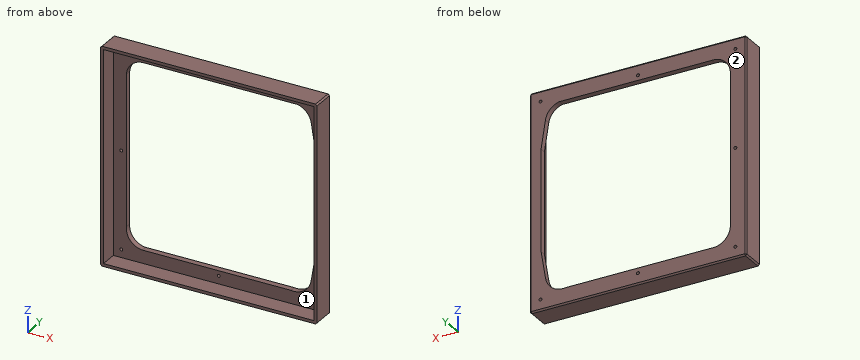
from build123d import *

# Parameters (mm, degrees)
SKETCH009_W     = 150
SKETCH009_H     = 150
SKETCH009_W_2   = 146
SKETCH009_H_2   = 146
PAD003_DEPTH    = 12
SKETCH010_W     = 150
SKETCH010_H     = 150
SKETCH010_R     = 1
PAD004_DEPTH    = 4
CHAMFER003_SIZE = 1


with BuildPart() as part:
    # Sketch009 → Pad003 (new body)
    with BuildSketch(Plane.XZ):
        Rectangle(SKETCH009_W, SKETCH009_H)
        Rectangle(SKETCH009_W_2, SKETCH009_H_2, mode=Mode.SUBTRACT)
    extrude(amount=PAD003_DEPTH)

    # Sketch010 (on Face9 of Pad003) → Pad004 (join)
    with BuildSketch(Plane(origin=(0, 0, 0), x_dir=(1, 0, 0), z_dir=(0, 1, 0))):
        Rectangle(SKETCH010_W, SKETCH010_H)
        with Locations((-67.5, 67.5)):
            Circle(SKETCH010_R, mode=Mode.SUBTRACT)
        with Locations((67.5, 67.5)):
            Circle(SKETCH010_R, mode=Mode.SUBTRACT)
        with Locations((0, 67.5)):
            Circle(SKETCH010_R, mode=Mode.SUBTRACT)
        with Locations((-67.5, 0)):
            Circle(SKETCH010_R, mode=Mode.SUBTRACT)
        with Locations((-67.5, -67.5)):
            Circle(SKETCH010_R, mode=Mode.SUBTRACT)
        with Locations((0, -67.5)):
            Circle(SKETCH010_R, mode=Mode.SUBTRACT)
        with Locations((67.5, -67.5)):
            Circle(SKETCH010_R, mode=Mode.SUBTRACT)
        with BuildLine():
            ThreePointArc((-53, 64), (-61.176409, 59.816751), (-64, 51.077152))
            Line((-64, 51.077152), (-64, -53))
            ThreePointArc((-64, -53), (-59.816751, -61.176409), (-51.077152, -64))
            Line((-51.077152, -64), (54.6127, -64))
            ThreePointArc((54.6127, -64), (60.907852, -60.466964), (64.115604, -54))
            Line((67.115604, -35), (64.115604, -54))
            Line((67.115604, 35), (67.115604, -35))
            Line((64, 54), (67.115604, 35))
            ThreePointArc((64, 54), (59.109644, 61.883516), (50.077152, 64))
            Line((50.077152, 64), (-53, 64))
        make_face(mode=Mode.SUBTRACT)
    extrude(amount=PAD004_DEPTH)

    # Chamfer003
    chamfer003_edges = [part.edges().sort_by_distance(p)[0] for p in [
        (0, 4, -75),
        (-75, 4, 0),
        (0, 4, 75),
        (75, 4, 0),
        (75, 2, -75),
        (75, -6, 75),
        (-75, -6, -75),
        (-75, -6, 75),
    ]]
    chamfer(chamfer003_edges, length=CHAMFER003_SIZE)


with BuildPart() as part_1:
    # Body001 placement: moved
    add(part.part.moved(Location((0, -3, 0))))


solid = part_1.part
Read the model definition and answer for the solid it produces. Units are mm, in the model's axes. Face numbers are marked on the shaded views. Round coordinates to 2 decimals unless told otherwise and drop trailing zeros. Write each loop counter-clockwise with the first axis right and the second up, starting at its lowest first coordinate (ties: lowest second). Pieces come first, ordered by that corner, then holes. Notation, with made-up numbers: (34, -7.5) - (74, -7.5) arc R20 ccw to (74, 5.5) - close; hole circle Ø5 at (-8, 83.5). An arc over 180 degrees is marked (long way). Use a Markdown table: item, result.
(1) The part is cut by section B-B (y = -11.5). Write down the section's boundary in (x, z).
Reported:
| item | result |
|---|---|
| outline | (-75, -74) - (-74, -75) - (74, -75) - (75, -74) - (75, 74) - (74, 75) - (-74, 75) - (-75, 74) - close; hole (-73, -73) - (73, -73) - (73, 73) - (-73, 73) - close |
(2) Each of these flat-tipped pins is pushed along its axis until it touches: pin 1 Ø1.2 at (x, z) = (67.5, 67.5) entering from +Y; pin 2 Ø2.5 at (x, z) = (0, -67.5) entering from +Y; pin 3 Ø3 at (x, z) = (-67.5, 67.5) entering from -Y. Where does it stop, or does it pass through?
Reported:
| item | result |
|---|---|
| pin 1 | through |
| pin 2 | y = 1 |
| pin 3 | y = -3 |
(3) The mould has two halves that part along Z. Classify the marked faces 1 and 2: released by +Z, released by -Z, zero draft, split by the parting line, or undercut.
Reported:
| item | result |
|---|---|
| face 1 | undercut |
| face 2 | zero draft |
(4) Straight lines are drawn through the part: line 1 along X through (y, z) = (-0.3, 67.5); line 2 along X through (y, z) = (-1.1, 0); line 3 along Z through (x, y) = (67.5, -0.75). For each, find the intervals that lie inside material, in ascending order. Write a range as [from, to].
Reported:
| item | result |
|---|---|
| line 1 | [-75, -68.5], [-66.5, -1], [1, 66.5], [68.5, 75] |
| line 2 | [-75, -68.5], [-66.5, -64], [67.12, 75] |
| line 3 | [-75, -68.5], [-66.5, 66.5], [68.5, 75] |
(5) The part is cut by section A-A (z = -29.5). Write down the section's boundary in (x, y).
Reported:
| item | result |
|---|---|
| outline | (-75, -15) - (-73, -15) - (-73, -3) - (-64, -3) - (-64, 1) - (-74, 1) - (-75, 0) - close; (67.12, -3) - (73, -3) - (73, -15) - (75, -15) - (75, 0) - (74, 1) - (67.12, 1) - close |
(6) The part is cut by section C-C (x = -6.5). Write down the section's boundary in (y, z).
Reported:
| item | result |
|---|---|
| outline | (-15, -75) - (0, -75) - (1, -74) - (1, -64) - (-3, -64) - (-3, -73) - (-15, -73) - close; (-15, 73) - (-3, 73) - (-3, 64) - (1, 64) - (1, 74) - (0, 75) - (-15, 75) - close |
